Build history of the part. All positions in model axes, mm. A direction names the side the tool comes from. Give positions to 0.01 mm unless a question says otherwise; leave off trailing zeros. Order: outer loops, then holes, each group sorted by start corner. A loop starts at its lowest first (then second) coordinate and runs counter-clockwise, first axis right, second up. Notation, with made-up numbers: M 40.5,56.25 L 99.5,56.25 A22 ccw 99.5,72.25 Z; hole C -13.75,-12.5 d9. An arc over 180 degrees is marked long. Answer as CSV lines item,"result".
Autodesk Inventor part; units mm, degrees
ref_plane "YZ Plane" through (0, 0, 0) normal (1, 0, 0) x (0, 1, 0)
ref_plane "XZ Plane" through (0, 0, 0) normal (0, 1, 0) x (-1, 0, 0)
ref_plane "XY Plane" through (0, 0, 0) normal (0, 0, 1) x (1, 0, 0)
sketch "Sketch1" plane through (0, 0, 0) normal (0, 1, 0) x (-1, 0, 0)
  line L0 (36.83, 24.13) -> (-36.83, 24.13)
  line L1 (-36.83, 24.13) -> (-36.83, -24.13)
  line L2 (-36.83, -24.13) -> (36.83, -24.13)
  line L3 (36.83, -24.13) -> (36.83, 24.13)
  line L4 (36.83, 24.13) -> (-36.83, -24.13) construction
  line L5 (-36.83, 24.13) -> (36.83, -24.13) construction
  line L6 (29.21, 20.32) -> (-29.21, 20.32)
  line L7 (-29.21, 20.32) -> (-29.21, -20.32)
  line L8 (-29.21, -20.32) -> (29.21, -20.32)
  line L9 (29.21, -20.32) -> (29.21, 20.32)
  line L10 (29.21, 20.32) -> (-29.21, -20.32) construction
  line L11 (-29.21, 20.32) -> (29.21, -20.32) construction
  point P0 (0, 0)
  dimension "d0" = 73.66
  dimension "d1" = 48.26
  dimension "d2" = 58.42
  dimension "d3" = 40.64
extrude "Extrusion1" add sketch "Sketch1" along normal blind 190.5
sketch "Sketch2" plane through (36.83, 0, 24.13) normal (1, 0, 0) x (0, 0, -1)
  line L0 (0, 0) -> (-10.16, 0)
  line L1 (48.26, 0) -> (48.26, 190.5)
  line L2 (48.26, 0) -> (58.42, 0)
  line L3 (-10.16, 0) -> (58.42, 0)
  line L4 (58.42, 0) -> (58.42, 190.5)
  line L5 (58.42, 190.5) -> (-10.16, 190.5)
  line L6 (-10.16, 190.5) -> (-10.16, 0)
  line L7 (-10.16, 190.5) -> (58.42, 190.5)
  line L8 (58.42, 190.5) -> (58.42, 200.66)
  line L9 (58.42, 200.66) -> (-10.16, 200.66)
  line L10 (-10.16, 200.66) -> (-10.16, 190.5)
  line L11 (0, 190.5) -> (48.26, 190.5)
  line L12 (-10.16, 0) -> (0, 0)
  line L13 (0, 0) -> (0, 190.5)
  line L14 (0, 190.5) -> (-10.16, 190.5)
  line L15 (-10.16, 190.5) -> (-10.16, 0)
  line L16 (0, 190.5) -> (58.42, 190.5)
  line L17 (58.42, 190.5) -> (58.42, 200.66)
  line L18 (58.42, 200.66) -> (0, 200.66)
  line L19 (0, 200.66) -> (0, 190.5)
  point P0 (24.13, 0)
  dimension "d6" = 10.16
  dimension "d7" = 10.16
  dimension "d8" = 10.16
extrude "Extrusion2" add sketch "Sketch2" against normal blind 90.5129 contours L1 L5 L4 L2 | L19 L9 L8 L5
extrude "Extrusion3" add sketch "Sketch2" along normal blind 16.8529 contours L1 L5 L4 L2 | L19 L9 L8 L5
sketch "Sketch3" plane through (-29.21, 190.5, 20.32) normal (0, -1, 0) x (1, 0, 0)
  line L0 (58.42, 0) -> (0, 0)
  line L1 (0, -40.64) -> (58.42, -40.64)
  line L2 (58.42, 0) -> (0, 0)
  line L3 (0, 0) -> (0, -40.64)
  line L4 (0, -40.64) -> (58.42, -40.64)
  line L5 (58.42, -40.64) -> (58.42, 0)
  line L6 (54.61, -3.81) -> (3.81, -3.81)
  line L7 (3.81, -3.81) -> (3.81, -36.83)
  line L8 (3.81, -36.83) -> (54.61, -36.83)
  line L9 (54.61, -36.83) -> (54.61, -3.81)
  line L10 (54.61, -3.81) -> (3.81, -36.83) construction
  line L11 (3.81, -3.81) -> (54.61, -36.83) construction
  point P0 (29.21, -20.32)
  dimension "d13" = 50.8
  dimension "d14" = 33.02
extrude "Extrusion4" cut sketch "Sketch3" against normal blind 10.16 contours L9 L8 L7 L6
properties part number "UE306_Sleeve"
Item 1: Band-saw the part on C-C (y = 181). Give the cut face in (x, z), and give its area (3 significant figures).
Geometry says:
outline,"M -53.68,-34.29 L 53.68,-34.29 L 53.68,-24.13 L 36.83,-24.13 L 36.83,24.13 L -36.83,24.13 L -36.83,-24.13 L -53.68,-24.13 Z; hole M -29.21,-20.32 L 29.21,-20.32 L 29.21,20.32 L -29.21,20.32 Z"
area,"2,270 mm2"
Item 2: Band-saw the part on D-D (x = -45). Give the cut face in (y, z).
Geometry says:
outline,"M 0,-34.29 L 200.66,-34.29 L 200.66,24.13 L 190.5,24.13 L 190.5,-24.13 L 0,-24.13 Z"
Item 3: Pull direction Z, two halves, no side cores. Call faces 4 (the flat face through (1, 200.66, -18)), 5 (the flat face through (29.21, 94, 0)), 6 (the flat face through (45, 94, -24.13)): released by +Z, released by -Z, zero draft, split by the parting line, or undercut.
Geometry says:
face 4,"zero draft"
face 5,"undercut"
face 6,"released by +Z"
Item 4: Probe line 1 along X through (y, z) = (170.5, 20); line 2 along Z through (x, y) = (22.5, 184.5); line 3 along Y through (x, z) = (41.5, -8.5). List the from-to ranges inside material, lowest first. Write a range as from..to.
Geometry says:
line 1,"x = -36.83..-29.21, 29.21..36.83"
line 2,"z = -34.29..-20.32, 20.32..24.13"
line 3,"y = 190.5..200.66"
Item 5: Band-saw the part on A-A (z = -8.5). Give the cut face in (x, y), and give its area (3 significant figures).
Geometry says:
outline,"M -53.68,190.5 L -36.83,190.5 L -36.83,0 L -29.21,0 L -29.21,190.5 L -25.4,190.5 L -25.4,200.66 L -53.68,200.66 Z; M 25.4,190.5 L 29.21,190.5 L 29.21,0 L 36.83,0 L 36.83,190.5 L 53.68,190.5 L 53.68,200.66 L 25.4,200.66 Z"
area,"3,480 mm2"
Item 6: Drop flat-ended pins along their axis: pin 1 (3 mm diameter, centred on y = 160.5, z = 18, fed in from -X); pin 2 (8.5 mm diameter, centred on x = -47, y = 113, fed in from +Z); pin 3 (8 mm diameter, centred on y = 93.5, z = -10.5, fed in from +X). Give the stop position or say it passes through.
Geometry says:
pin 1,"stops at x = -36.83"
pin 2,"stops at z = -24.13"
pin 3,"stops at x = 36.83"
Item 7: 3-axis set-ups, long thin cutter, end or side, ignore diameter. For faces 1 (the flat face through (0, 190.5, -18)), 2 (the flat face through (0, 196, -16.51)), 3 (the flat face through (45, 190.5, 0)): which of +Z, -Z, +X, -X, +Y, -Y reach the whole face in a straight line?
Geometry says:
face 1,"-Y"
face 2,"+Y, -Y"
face 3,"+Z, +X, -Y"
Item 8: Band-saw the part on B-B (x = 16.5). Give the cut face in (y, z).
Geometry says:
outline,"M 0,-34.29 L 200.66,-34.29 L 200.66,-16.51 L 190.5,-16.51 L 190.5,-20.32 L 0,-20.32 Z; M 0,20.32 L 190.5,20.32 L 190.5,16.51 L 200.66,16.51 L 200.66,24.13 L 0,24.13 Z"
